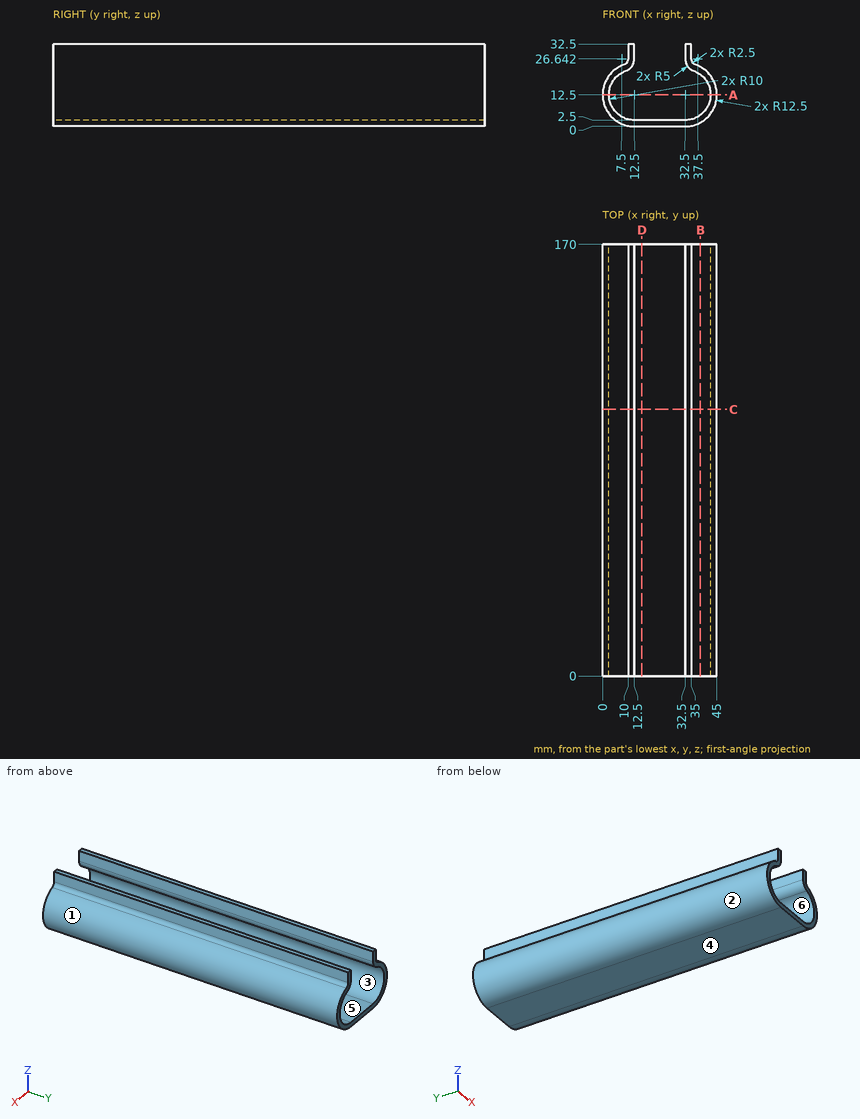
Verification items for this drawing (mm, ordinates from the low corner). A direction names the side the tool comes from. Coordinates: 2 decimals unless noted, no trailing zeros. Order: outer loops, then holes, each group sorted by start corner. A loop starts at its lowest first (then second) coordinate and runs counter-clockwise, first axis right, second up. Notation, with made-up numbers: (69.5, -39.75) - (106.5, -39.75) arc R11 cw to (106.5, -26.75) - close; hole circle Ø11 at (34.25, 35.25). An arc over 180 degrees is marked (long way). Answer in a Markdown table with one row per item. Add a question column.
1. Section check C-C (y = 105). Enter the section's corners in (x, z) (1 decimal).
2. Section check B-B (x = 38.5). Enter the section's corners in (y, z), plus the area to 3 significant figures.
3. Section check D-D (x = 15.5). Enter the section's corners in (y, z), plus the area to 3 significant figures.
4. Access from +Z, -Z, +X, -X, +Y, -Y to the whole of each face (thin tool, end or side, straight path). Record for the marked faces 5 and 6.
5. Material ranges on L1, parallel to X at y = 45, z = 26.5; L2, parallel to X at y = 16, z = 13; L3, parallel to Z at x = 32, y = 119, recorded low to high. Write a range as [from, to].
6. Draft check along X on the marked faces 1, 2, 3 and 4. Enter one of: +X half, -X half, draft (parallel to the pull), parting line (faces both ways), or undercut.
7. Gauge pin test, flat ends, axial feed: pin 1 Ø3 at (y, z) = (67, 30.5) entering from +X; pin 2 Ø16 at (x, y) = (21, 85) entering from +Z; pin 3 Ø6 at (y, z) = (122.5, 24.5) entering from -X (1 decimal). Record the tip position at first contact, or that the pin passes through.
8. Section check A-A (z = 12.5). Enter the section's corners in (x, y), plus the area to 3 significant figures.
Data:
| question | item | result |
|---|---|---|
| 1 | outline | (8.3, 24.3) arc R12.5 ccw to (12.5, 0) - (32.5, 0) arc R12.5 ccw to (36.7, 24.3) arc R2.5 cw to (35, 26.6) - (35, 32.5) - (32.5, 32.5) - (32.5, 26.6) arc R5 ccw to (35.8, 21.9) arc R10 cw to (32.5, 2.5) - (12.5, 2.5) arc R10 cw to (9.2, 21.9) arc R5 ccw to (12.5, 26.6) - (12.5, 32.5) - (10, 32.5) - (10, 26.6) arc R2.5 cw to start |
| 2 | outline | (0, 1.53) - (170, 1.53) - (170, 4.5) - (0, 4.5) - close; (0, 20.5) - (170, 20.5) - (170, 23.47) - (0, 23.47) - close |
| 2 | area | 1,010 mm² |
| 3 | outline | (0, 0) - (170, 0) - (170, 2.5) - (0, 2.5) - close |
| 3 | area | 425 mm² |
| 4 | face 5 | +Z, +Y, -Y |
| 4 | face 6 | +Y, -Y |
| 5 | L1 | x = [10, 12.5], [32.5, 35] |
| 5 | L2 | x = [0.01, 2.51], [42.49, 44.99] |
| 5 | L3 | z = [0, 2.5] |
| 6 | face 1 | +X half |
| 6 | face 2 | -X half |
| 6 | face 3 | undercut |
| 6 | face 4 | draft |
| 7 | pin 1 | stops at x = 35 |
| 7 | pin 2 | stops at z = 2.5 |
| 7 | pin 3 | stops at x = 3.8 |
| 8 | outline | (0, 0) - (2.5, 0) - (2.5, 170) - (0, 170) - close; (42.5, 0) - (45, 0) - (45, 170) - (42.5, 170) - close |
| 8 | area | 850 mm² |
